Read the model definition and answer for the solid it produces. Units are mm, in the model's axes. Coordinates: 2 decimals unless noted, no trailing zeros. Write each loop counter-clockwise with the first axis right and the second up, starting at its lowest first coordinate (ties: lowest second). Pieces come first, ordered by that corner, then holes.
(1) Given pin 1 (10 mm diameter, centred on y = 23.5, z = 23.5, fed in from +X); pin 2 (2 mm diameter, centred on x = 21.5, z = 33.5, fed in from +Y); pin 3 (3 mm diameter, centred on y = 21, z = -21.5, fed in from -X), each flat-ended and moving along its own axis, determine where each tip first touches the part or whether it passes through.
(2) Straight lines are drawn through the part: line 1 along Z through (x, y) = (-58, -25); line 2 along Z through (x, y) = (-46, -12.5); line 3 along Y through (x, z) = (-11, 0.5). For each, find the intervals that lie inside material, in ascending order.
(3) The part is cut by section A-A, the plane z = 0. Determine the outline of the cut face in (x, y) (3 decimals).
```python
from build123d import *

# Parameters (mm, degrees)
F1_R     = 6.35
F2_DEPTH = 66.04
F4_R     = 9.525
F5_DEPTH = 64.77


with BuildPart() as f2:
    # F1 (on Right) → F2 (new body)
    with BuildSketch(Plane.YZ):
        Circle(F1_R)
    extrude(amount=F2_DEPTH)

    # F0 (on Front) → F3 (revolve)
    with BuildSketch(Plane.XZ):
        with BuildLine():
            Line((0, 12.7), (0, 63.5))
            ThreePointArc((0, 63.5), (-40.160926, 49.186888), (-62.217039, 12.7))
            Line((-62.217039, 12.7), (-60.090102, 12.7))
            Line((-60.090102, 12.7), (0, 12.7))
        make_face()
        Polygon((-60.090102, 12.7), (-62.217039, 12.7), (-64.71397, 12.7), (-64.548267, 10.621531), (-60.090102, 10.621531), align=None)
        Polygon((0, -12.7), (0, 12.7), (-60.090102, 12.7), (-60.090102, 10.621531), (-60.090102, -10.621531), (-60.090102, -12.7), align=None)
        with BuildLine():
            Line((0, -63.5), (0, -12.7))
            Line((0, -12.7), (-60.090102, -12.7))
            Line((-60.090102, -12.7), (-62.217039, -12.7))
            ThreePointArc((-62.217039, -12.7), (-40.160926, -49.186888), (0, -63.5))
        make_face()
        Polygon((-62.217039, -12.7), (-60.090102, -12.7), (-60.090102, -10.621531), (-64.548267, -10.621531), (-64.71397, -12.7), align=None)
    revolve(axis=Axis((0, 0, 0), (0, 0, -1)))

    # F4 (on Right) → F5 (join)
    with BuildSketch(Plane.YZ):
        Circle(F4_R)
    extrude(amount=F5_DEPTH)


solid = f2.part
```
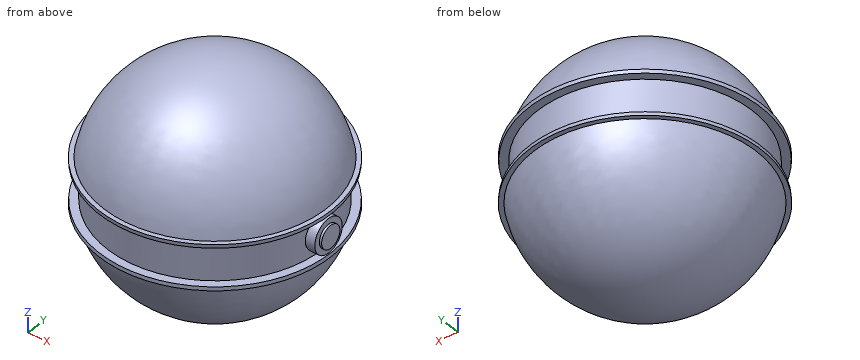
Computed:
1. pin 1: stops at x = 56.88
1. pin 2: stops at y = 50.26
1. pin 3: stops at x = -56.72
2. line 1: z = -12.7 to -10.62, 10.62 to 12.7
2. line 2: z = -41.95 to 41.95
2. line 3: y = -59.07 to 59.07
3. outline: (59.33, -9.525) - (64.77, -9.525) - (64.77, -6.35) - (66.04, -6.35) - (66.04, 6.35) - (64.77, 6.35) - (64.77, 9.525) - (59.33, 9.525) arc R60.09 ccw (long way) to start
